Model file for the job. Use its own axes, mm. Face numbers are marked on the shaded views. A direction names the side the tool comes from. Round coordinates to 2 decimals unless told otherwise and drop trailing zeros. Loops run counter-clockwise (first coordinate to the right, second up) from the corner with the lowest first, then second, coordinate; pieces in that order, holes last.
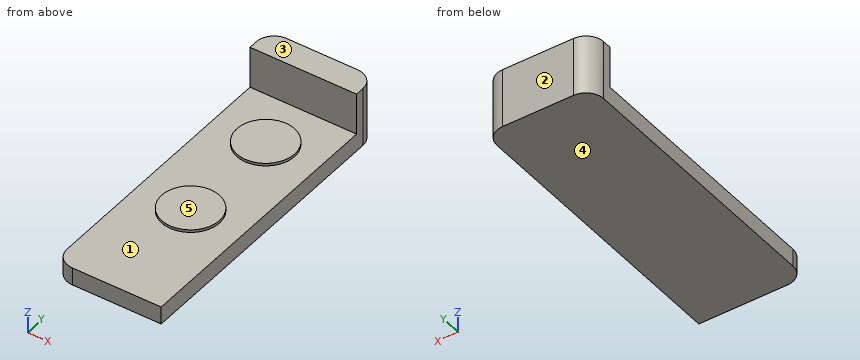
from build123d import *

# Parameters (mm, degrees)
ESQUISSE1_W        = 12
ESQUISSE1_H        = 34.2
BOSS_EXTRU_1_DEPTH = 2
ESQUISSE2_R        = 3.25
BOSS_EXTRU_2_DEPTH = 0.3
ESQUISSE3_W        = 12
ESQUISSE3_H        = 3
BOSS_EXTRU_3_DEPTH = 4.7
CONG_1_R           = 2


with BuildPart() as part:
    # Esquisse1 → Boss.-Extru.1 (new body)
    with BuildSketch(Plane.XY):
        with Locations((2.233800948, 3.291549296)):
            Rectangle(ESQUISSE1_W, ESQUISSE1_H)
    extrude(amount=BOSS_EXTRU_1_DEPTH)

    # Esquisse2 → Boss.-Extru.2 (add)
    with BuildSketch(Plane.XY.offset(2)):
        with Locations((2.233800948, 11.391549296)):
            Circle(ESQUISSE2_R)
        with Locations((2.233800948, -0.608450704)):
            Circle(ESQUISSE2_R)
    extrude(amount=BOSS_EXTRU_2_DEPTH)

    # Esquisse3 → Boss.-Extru.3 (add)
    with BuildSketch(Plane.XY.offset(2)):
        with Locations((2.233800948, 18.891549296)):
            Rectangle(ESQUISSE3_W, ESQUISSE3_H)
    extrude(amount=BOSS_EXTRU_3_DEPTH)

    # Congé1
    cong_1_edges = [part.edges().sort_by_distance(p)[0] for p in [
        (-3.766199052, 20.391549296, 3.35),
        (8.233800948, 20.391549296, 3.35),
        (-3.766199052, -13.808450704, 1),
    ]]
    fillet(cong_1_edges, radius=CONG_1_R)


solid = part.part
Q1. Slice it at C-C on x = 2.25. Give the cut face in (y, z).
Q2. Probe line 1 (Y direction, x = 1.5, z = 3); line 2 (Z direction, x = -1.5, y = 9); line 3 (Z direction, x = -0.75, y = 12). List the from-to ranges inside material, lowest first.
Q3. Flat gauge pins, fed straight in: P1, Ø5, axis at x = 0.5, y = 4, coming from the +Z side; P2, Ø4, axis at x = 4, z = 5.5, coming from the -Y side. Where does each tip first touch, or does it go through?
Q4. Pull direction Y, two halves, no side cores. Call the marked faces 1, 2 and 3: pulls with the +Y half, pulls with the -Y half, needs draft (parallel to the pull), parting line crosses it, or undercut.
Q5. Slice it at D-D on y = 12. Give the cut face in (x, z).
Q6. Slice it at B-B on z = 2.75. Give the cut face in (x, y), plus the area to 3 significant figures.
Q7. Slice it at A-A on y = 8.5. Give the cut face in (x, z).
Q8. Tool access for the marked faces 4 and 5: list every direction of +Z, -Z, +X, -X, +Y, -Y with a clear straight run to the whole face (end or side of a thin tool).
Reply:
1. outline: (-13.81, 0) - (20.39, 0) - (20.39, 6.7) - (17.39, 6.7) - (17.39, 2) - (14.64, 2) - (14.64, 2.3) - (8.14, 2.3) - (8.14, 2) - (2.64, 2) - (2.64, 2.3) - (-3.86, 2.3) - (-3.86, 2) - (-13.81, 2) - close
2. line 1: y = 17.39 to 20.39
2. line 2: z = 0 to 2
2. line 3: z = 0 to 2.3
3. P1: stops at z = 2.3
3. P2: stops at y = 17.39
4. face 1: undercut
4. face 2: pulls with the +Y half
4. face 3: needs draft
5. outline: (-3.77, 0) - (8.23, 0) - (8.23, 2) - (5.43, 2) - (5.43, 2.3) - (-0.96, 2.3) - (-0.96, 2) - (-3.77, 2) - close
6. outline: (-3.77, 17.39) - (8.23, 17.39) - (8.23, 18.39) arc R2 ccw to (6.23, 20.39) - (-1.77, 20.39) arc R2 ccw to (-3.77, 18.39) - close
6. area: 34.3 mm2
7. outline: (-3.77, 0) - (8.23, 0) - (8.23, 2) - (3.72, 2) - (3.72, 2.3) - (0.75, 2.3) - (0.75, 2) - (-3.77, 2) - close
8. face 4: -Z, +X, -X, +Y, -Y
8. face 5: +Z, +X, -X, -Y
